For this review, take the finished solid that the model builds, in its own axes (mm). Face numbers are marked on the shaded views. A direction names the side the tool comes from. Coordinates: 2 decimals unless noted, no trailing zeros. Write each loop counter-clockwise with the first axis right and the second up, starting at its lowest first coordinate (ties: lowest second). Pieces come first, ordered by that corner, then holes.
1) We need section C-C on y = 23. Write out the cut boundary in (x, z).
2) We need section A-A on x = 28.25. Write out the cut boundary in (y, z), then the cut area to 3 significant figures.
3) For the marked faces 4 and 5, list the 3-axis set-ups (+Z, -Z, +X, -X, +Y, -Y) from which the entire face can be reached by the end or side of a thin tool; tool diameter is ignored.
4) Mouldability with a two-part tool opening along X and no side actions: class the marked faces 1, 2 and 3 as pulls with the +X half, pulls with the -X half, needs draft (parallel to the pull), parting line crosses it, or undercut.
5) Insertion check: P1, Ø12, axis at y = 11.5, z = 14.5, coming from the -X side; P2, Ø1.9, axis at x = 28.25, y = 8, coming from the -Z side; P3, Ø2.5, axis at x = -30, y = 25.5, coming from the +Z side; P4, Ø4, axis at x = -26, y = 9.5, coming from the +Z side. Each pin has a flat end and moves straight along its axis. Give the tip position at first contact, or say it passes through.
6) We need section D-D on x = 0. Write out the cut boundary in (y, z), then the cut area to 3 significant figures.
7) To check wall thickness, follow line 1 along Y through (x, z) = (28.25, 2.45); line 2 along Z through (x, y) = (30.5, 6); line 3 along Z through (x, y) = (-11.5, 36). State the ranges of each line that lie inside material, in increasing order.
8) We need section B-B on y = 8. Write out the cut boundary in (x, z).
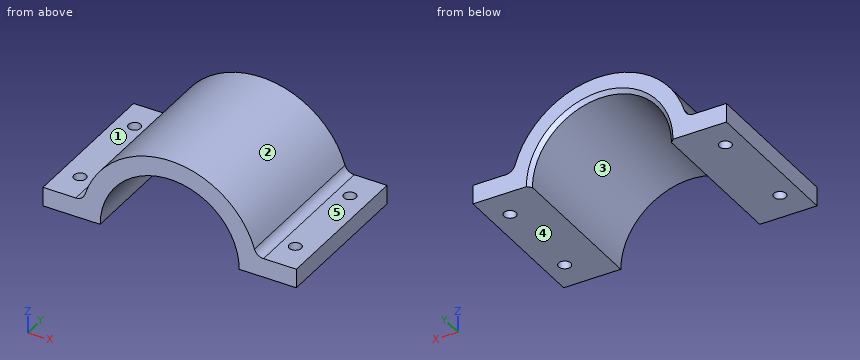
from build123d import *

# Parameters (mm, degrees)
EXTRUDE_1_DEPTH     = 40.25
SKETCH_2_W          = 10
SKETCH_2_H          = 40.25
EXTRUDE_2_DEPTH     = 5
EXTRUDE_2_2_DEPTH   = 5
EXTRUDE_3_DEPTH     = 40.25
CHAMFER_1_SIZE      = 1
SKETCH_4_R          = 1.6
CUT_EXTRUDE_1_DEPTH = 24.25


with BuildPart() as part:
    # Sketch 1 → Extrude 1 (new body)
    with BuildSketch(Plane(origin=(0, 0, 0), x_dir=(1, 0, 0), z_dir=(0, 1, 0))):
        with BuildLine():
            Line((-23.25, 0), (-18.25, 0))
            ThreePointArc((-18.25, 0), (0, -18.25), (18.25, 0))
            Line((18.25, 0), (23.25, 0))
            ThreePointArc((23.25, 0), (0, -23.25), (-23.25, 0))
        make_face()
    extrude(amount=EXTRUDE_1_DEPTH)



with BuildPart() as body_2:
    # Sketch 2 → Extrude 2 (new body)
    with BuildSketch(Plane(origin=(0, 0, 0), x_dir=(-1, 0, 0), z_dir=(0, 0, -1))):
        with Locations((-28.25, 20.125)):
            Rectangle(SKETCH_2_W, SKETCH_2_H)
    extrude(amount=-EXTRUDE_2_DEPTH)


with BuildPart() as body_3:
    # Sketch 2 → Extrude 2 2 (new body)
    with BuildSketch(Plane(origin=(0, 0, 0), x_dir=(-1, 0, 0), z_dir=(0, 0, -1))):
        with Locations((28.25, 20.125)):
            Rectangle(SKETCH_2_W, SKETCH_2_H)
    extrude(amount=-EXTRUDE_2_2_DEPTH)


with BuildPart() as part_1:
    add(part.part)

    add(body_2.part)  # Extrude 3 merges body 2

    add(body_3.part)  # Extrude 3 merges body 3
    # Sketch 3 → Extrude 3 (add)
    with BuildSketch(Plane(origin=(0, 40.25, 0), x_dir=(1, 0, 0), z_dir=(0, 1, 0))):
        with BuildLine():
            Line((23.25, -5), (23.25, 0))
            ThreePointArc((23.25, 0), (22.996608271, -3.423230646), (22.241956297, -6.77184466))
            ThreePointArc((22.241956297, -6.77184466), (23.14534213, -5.491220725), (24.6335645, -5))
            Line((24.6335645, -5), (23.25, -5))
        make_face()
        with BuildLine():
            Line((-23.25, -5), (-23.25, 0))
            ThreePointArc((-23.25, 0), (-22.996608271, -3.423230646), (-22.241956297, -6.77184466))
            ThreePointArc((-22.241956297, -6.77184466), (-23.14534213, -5.491220725), (-24.6335645, -5))
            Line((-24.6335645, -5), (-23.25, -5))
        make_face()
    extrude(amount=-EXTRUDE_3_DEPTH)

    # Chamfer 1
    chamfer_1_edges = [part_1.edges().sort_by_distance(p)[0] for p in [
        (0, 40.25, 18.25),
    ]]
    chamfer(chamfer_1_edges, length=CHAMFER_1_SIZE)

    # Sketch 4 → Cut-Extrude 1 (cut, through all)
    with BuildSketch(Plane(origin=(0, 0, 0), x_dir=(-1, 0, 0), z_dir=(0, 0, -1))):
        with Locations((28.25, 32.25)):
            Circle(SKETCH_4_R)
        with Locations((28.25, 8)):
            Circle(SKETCH_4_R)
        with Locations((-28.25, 32.25)):
            Circle(SKETCH_4_R)
        with Locations((-28.25, 8)):
            Circle(SKETCH_4_R)
    extrude(amount=-CUT_EXTRUDE_1_DEPTH, mode=Mode.SUBTRACT)


solid = part_1.part
Result:
1. outline: (-33.25, 0) - (-18.25, 0) arc R18.25 cw to (18.25, 0) - (33.25, 0) - (33.25, 5) - (24.63, 5) arc R2.5 cw to (22.24, 6.77) arc R23.25 ccw to (-22.24, 6.77) arc R2.5 cw to (-24.63, 5) - (-33.25, 5) - close
2. outline: (0, 0) - (6.4, 0) - (6.4, 5) - (0, 5) - close; (9.6, 0) - (30.65, 0) - (30.65, 5) - (9.6, 5) - close; (33.85, 0) - (40.25, 0) - (40.25, 5) - (33.85, 5) - close
2. area: 169 mm2
3. face 4: -Z, +X, -X, +Y, -Y
3. face 5: +Z, +X, +Y, -Y
4. face 1: needs draft
4. face 2: parting line crosses it
4. face 3: undercut
5. P1: stops at x = -21.64
5. P2: passes through
5. P3: stops at z = 5
5. P4: stops at z = 5.08
6. outline: (0, 18.25) - (39.25, 18.25) - (40.25, 19.25) - (40.25, 23.25) - (0, 23.25) - close
6. area: 201 mm2
7. line 1: y = 0 to 6.4, 9.6 to 30.65, 33.85 to 40.25
7. line 2: z = 0 to 5
7. line 3: z = 14.17 to 20.21
8. outline: (-33.25, 0) - (-29.85, 0) - (-29.85, 5) - (-33.25, 5) - close; (-26.65, 0) - (-18.25, 0) arc R18.25 cw to (18.25, 0) - (26.65, 0) - (26.65, 5) - (24.63, 5) arc R2.5 cw to (22.24, 6.77) arc R23.25 ccw to (-22.24, 6.77) arc R2.5 cw to (-24.63, 5) - (-26.65, 5) - close; (29.85, 0) - (33.25, 0) - (33.25, 5) - (29.85, 5) - close
